```python
from build123d import *

# Parameters (mm, degrees)
F0_R     = 10.414
F1_DEPTH = 1.6
F2_R     = 8.89
F3_DEPTH = 3.175
F4_R     = 1.856091
F4_R_2   = 1.80108
F4_R_3   = 1.799605
F5_DEPTH = 1.1938
F6_W     = 2.8
F6_H     = 3.1
F7_DEPTH = 0.6


with BuildPart() as f1:
    # F0 (on Top) → F1 (new body)
    with BuildSketch(Plane.XY):
        Circle(F0_R)
    extrude(amount=F1_DEPTH)

    # F2 (on face) → F3 (join)
    with BuildSketch(Plane(origin=(0, 0, 0), x_dir=(1, 0, 0), z_dir=(0, 0, -1))):
        Circle(F2_R)
    extrude(amount=F3_DEPTH)

    # F4 (on face) → F5 (join)
    with BuildSketch(Plane.XY.offset(1.6)):
        with Locations((0, 5.588)):
            Circle(F4_R)
        with Locations((3.556, -4.318)):
            Circle(F4_R_2)
        with Locations((-6.858, 0.508)):
            Circle(F4_R_3)
    extrude(amount=F5_DEPTH)

    # F6 (on face) → F7 (join)
    with BuildSketch(Plane.XY.offset(1.6)):
        with Locations((-0.003, 0.0006)):
            Rectangle(F6_W, F6_H)
    extrude(amount=F7_DEPTH)


solid = f1.part
```
Build history of the part. All positions in model axes, mm. A direction names the side the tool comes from. Round coordinates to 2 decimals unless told otherwise and drop trailing zeros. Loops run counter-clockwise (first coordinate to the right, second up) from the corner with the lowest first, then second, coordinate; pieces in that order, holes last. Notation, with made-up numbers: M -39.5,45.5 L 14.5,45.5 A20 ccw 14.5,54.5 Z; hole C 39,-9.5 d6. An arc over 180 degrees is marked long. Answer as CSV lines item,"result".
1. Cut at B-B on x = 0. Write the cut outline in (y, z) (3 decimals), then the cut area to 3 significant figures.
Resolved:
outline,"M -10.414,0 L -8.89,0 L -8.89,-3.175 L 8.89,-3.175 L 8.89,0 L 10.414,0 L 10.414,1.6 L 7.444,1.6 L 7.444,2.794 L 3.732,2.794 L 3.732,1.6 L 1.551,1.6 L 1.551,2.2 L -1.549,2.2 L -1.549,1.6 L -10.414,1.6 Z"
area,"96.1 mm²"
2. Two-plate mould, pull along Y, no slides. Class faces 1 (the flat face through (-7, 1, 2.794)), 2 (the cylindrical face through (-0.402, 3.776, 2.189)), 3 (the cylindrical face through (-8.286, -0.587, 2.189)): released by +Y, released by -Y, zero draft, split by the parting line, or undercut.
Resolved:
face 1,"zero draft"
face 2,"undercut"
face 3,"split by the parting line"
3. 3-axis set-ups, long thin cutter, end or side, ignore diameter. For faces 4 (the cylindrical face through (-1.93, 8.68, -1.57)), 5 (the flat face through (4, -4, 2.794)), 6 (the cylindrical face through (3.322, -2.532, 2.189)), 7 (the flat face through (0, 0, 2.2)): which of +Z, -Z, +X, -X, +Y, -Y reach the whole face in a straight line?
Resolved:
face 4,"-Z"
face 5,"+Z, +X, -X, +Y, -Y"
face 6,"+Z"
face 7,"+Z, +X, -Y"
4. Flat gauge pins, fed straight in: P1, Ø5, axis at x = -6.5, y = -4, coming from the +Z side; P2, Ø1.4, axis at x = 0, y = -1, coming from the +Z side; P3, Ø0.5, axis at y = -0.5, z = 2, coming from the -X side. Where does each tip first touch, or does it go through?
Resolved:
P1,"stops at z = 1.6"
P2,"stops at z = 2.2"
P3,"stops at x = -8.49"
5. Cut at C-C on z = 1.3. Write the cut outline in (x, y).
Resolved:
outline,"C 0,0 d20.83"
6. Cut at A-A on y = -5.5. Write the cut outline in (x, z) (3 decimals), then the cut area to 3 significant figures.
Resolved:
outline,"M -8.843,0 L -6.984,0 L -6.984,-3.175 L 6.984,-3.175 L 6.984,0 L 8.843,0 L 8.843,1.6 L 4.915,1.6 L 4.915,2.794 L 2.197,2.794 L 2.197,1.6 L -8.843,1.6 Z"
area,"75.9 mm²"
7. Cut at D-D on y = 6. Write the cut outline in (x, z) (3 decimals), then the cut area to 3 significant figures.
Resolved:
outline,"M -8.512,0 L -6.56,0 L -6.56,-3.175 L 6.56,-3.175 L 6.56,0 L 8.512,0 L 8.512,1.6 L 1.81,1.6 L 1.81,2.794 L -1.81,2.794 L -1.81,1.6 L -8.512,1.6 Z"
area,"73.2 mm²"
8. Wall check: probe 1 along Z at (x, y) = (-0.25, -1.5) (3 decimals); probe 2 along Z at (x, y) = (4.5, -0.25) (3 decimals); probe 3 along X at (y, z) = (0, -2.2). Give the ranges that are in metal, low to high. Write a range as [from, to].
Resolved:
probe 1,"z = [-3.175, 2.2]"
probe 2,"z = [-3.175, 1.6]"
probe 3,"x = [-8.89, 8.89]"
